Source: CAD feature listing. Evaluate the final solid. Frame: model axes, mm. A direction names the side the tool comes from. Give positions to 0.01 mm unless a question says otherwise; leave off trailing zeros. Loops run counter-clockwise (first coordinate to the right, second up) from the corner with the lowest first, then second, coordinate; pieces in that order, holes last. Notation, with made-up numbers: (-34, -32) - (-27, -32) arc R20 ccw to (-27, -19) - close; hole circle Ø3 at (11.25, 80). An arc over 180 degrees is marked (long way). Write each question's results on one line, items separated by ' | '. Start each with the question number.
(1) Cut plane C-C on x = -12. Return the cut outline in (y, z), then the cut area to 3 significant figures.
(2) Cut plane B-B on z = -73. Return the cut outline in (x, y), then the cut area to 3 significant figures.
(3) Material intervals for line 1 along Z through (x, y) = (52, 5.45); line 2 along X through (y, z) = (4.45, -70); line 3 along X through (y, z) = (2.6, -5), sorted ascending. Write a range as [from, to].
(4) Contact query for flat-ended pins moving along their axis: pin 1 (3 mm diameter, centred on x = 19, z = -70, fed in from -Y); pin 2 (1.8 mm diameter, centred on x = -12.5, y = 3, fed in from +Z); pin 3 (1.8 mm diameter, centred on y = 3.5, z = -12.5, fed in from -X); pin 4 (13 mm diameter, centred on x = -14, z = -51, fed in from -Y). Output: stop coordinate, or through.
(5) Cut plane A-A on x = 10. Return the cut outline in (y, z), then the cut area to 3 significant figures.
(6) Cut plane D-D on y = 1.1. Return the cut outline in (x, z).
(7) Reachability of faces 1 (the flat face through (40, 3, -19)), 2 (the flat face through (0, 3, -19)), 3 (the flat face through (-13, 3, -60)) from +Z, -Z, +X, -X, +Y, -Y: full face, straight path, thin tool, end or side. Return the list, or none.
(8) Pull-direction query (Z, two-part tool) for faces 4 (the cylindrical face through (11.054, 2.958, -50.672)), 5 (the flat face through (20, 3, 0)), 6 (the cylindrical face through (30.38, 2.96, -71.19)), 7 (the flat face through (21, 3, -80)); classes: pulls with the +Z half, pulls with the -Z half, needs draft (parallel to the pull), parting line crosses it, or undercut.
from build123d import *

# Parameters (mm, degrees)
EXTRUDE_1_DEPTH     = 6
FILLET_1_R          = 2
SKETCH_18_W         = 12
SKETCH_18_H         = 40
CUT_EXTRUDE_7_DEPTH = 3
SKETCH_19_R         = 1.5
CUT_EXTRUDE_8_DEPTH = 10
SKETCH_20_R         = 1.25
CUT_EXTRUDE_9_DEPTH = 10


with BuildPart() as part:
    # 草图1 → 凸台-拉伸1 (new body)
    with BuildSketch(Plane(origin=(0, 0, 0), x_dir=(1, 0, 0), z_dir=(0, 1, 0))):
        Polygon((0, 0), (40, 0), (40, 40), (59, 40), (59, 80), (-19, 80), (-19, 40), (0, 40), align=None)
    extrude(amount=EXTRUDE_1_DEPTH)

    # 圆角1
    fillet_1_edges = [part.edges().sort_by_distance(p)[0] for p in [
        (0, 3, -40),
        (40, 3, -40),
    ]]
    fillet(fillet_1_edges, radius=FILLET_1_R)

    # 草图18 → 切除-拉伸7 (cut)
    with BuildSketch(Plane.XZ):
        with Locations((-13, -60)):
            Rectangle(SKETCH_18_W, SKETCH_18_H)
        with Locations((53, -60)):
            Rectangle(SKETCH_18_W, SKETCH_18_H)
    extrude(amount=-CUT_EXTRUDE_7_DEPTH, mode=Mode.SUBTRACT)

    # 草图19 → 切除-拉伸8 (cut)
    with BuildSketch(Plane.XZ.offset(-3)):
        with Locations(Location((-12, -48, 0), (0, 0, 270))):
            Circle(SKETCH_19_R)
        with Locations(Location((-12, -73, 0), (0, 0, 270))):
            Circle(SKETCH_19_R)
        with Locations(Location((52, -73, 0), (0, 0, 90))):
            Circle(SKETCH_19_R)
        with Locations(Location((52, -48, 0), (0, 0, 90))):
            Circle(SKETCH_19_R)
    extrude(amount=-CUT_EXTRUDE_8_DEPTH, mode=Mode.SUBTRACT)

    # 草图20 → 切除-拉伸9 (cut)
    with BuildSketch(Plane.XZ):
        with Locations(Location((10, -5, 0), (0, 0, 270))):
            Circle(SKETCH_20_R)
        with Locations(Location((30, -5, 0), (0, 0, 270))):
            Circle(SKETCH_20_R)
        with Locations(Location((10, -50, 0), (0, 0, 270))):
            Circle(SKETCH_20_R)
        with Locations(Location((10, -70, 0), (0, 0, 270))):
            Circle(SKETCH_20_R)
        with Locations(Location((30, -50, 0), (0, 0, 270))):
            Circle(SKETCH_20_R)
        with Locations(Location((30, -70, 0), (0, 0, 270))):
            Circle(SKETCH_20_R)
    extrude(amount=-CUT_EXTRUDE_9_DEPTH, mode=Mode.SUBTRACT)


solid = part.part
Ans:
1) outline: (3, -80) - (6, -80) - (6, -74.5) - (3, -74.5) - close; (3, -71.5) - (6, -71.5) - (6, -49.5) - (3, -49.5) - close; (3, -46.5) - (6, -46.5) - (6, -40) - (3, -40) - close | area: 102 mm^2
2) outline: (-19, 3) - (-13.5, 3) - (-13.5, 6) - (-19, 6) - close; (-10.5, 3) - (-7, 3) - (-7, 0) - (47, 0) - (47, 3) - (50.5, 3) - (50.5, 6) - (-10.5, 6) - close; (53.5, 3) - (59, 3) - (59, 6) - (53.5, 6) - close | area: 378 mm^2
3) line 1: [-80, -74.5], [-71.5, -49.5], [-46.5, -40] | line 2: [-19, 8.75], [11.25, 28.75], [31.25, 59] | line 3: [0, 8.75], [11.25, 28.75], [31.25, 40]
4) pin 1: y = 0 | pin 2: z = -40 | pin 3: x = 0 | pin 4: y = 3
5) outline: (0, -80) - (6, -80) - (6, -71.25) - (0, -71.25) - close; (0, -68.75) - (6, -68.75) - (6, -51.25) - (0, -51.25) - close; (0, -48.75) - (6, -48.75) - (6, -6.25) - (0, -6.25) - close; (0, -3.75) - (6, -3.75) - (6, 0) - (0, 0) - close | area: 435 mm^2
6) outline: (-7, -80) - (47, -80) - (47, -40) - (42, -40) arc R2 cw to (40, -38) - (40, 0) - (0, 0) - (0, -38) arc R2 cw to (-2, -40) - (-7, -40) - close; hole circle Ø2.5 at (10, -70); hole circle Ø2.5 at (10, -50); hole circle Ø2.5 at (10, -5); hole circle Ø2.5 at (30, -70); hole circle Ø2.5 at (30, -50); hole circle Ø2.5 at (30, -5)
7) face 1: +Z, +X, +Y, -Y | face 2: +Z, -X, +Y, -Y | face 3: +Z, -Z, -X, -Y
8) face 4: undercut | face 5: pulls with the +Z half | face 6: undercut | face 7: pulls with the -Z half
